```python
from build123d import *

# Parameters (mm, degrees)
CYLINDER062_R     = 1.25
CYLINDER062_DEPTH = 5
CYLINDER038_R     = 3
CYLINDER038_DEPTH = 4.1


with BuildPart() as b_w009:
    # Cylinder062 → Cylinder062 (new body)
    with BuildSketch(Plane(origin=(2, 6, 26), x_dir=(0, 0, 1), z_dir=(-1, 0, 0))):
        Circle(CYLINDER062_R)
    extrude(amount=CYLINDER062_DEPTH)


with BuildPart() as cut023:
    # Cylinder038 → Cylinder038 (new body)
    with BuildSketch(Plane(origin=(-1, 6, 26), x_dir=(0, 0, -1), z_dir=(1, 0, 0))):
        Circle(CYLINDER038_R)
    extrude(amount=CYLINDER038_DEPTH)

    # Cut023: cut B_W009
    add(b_w009.part, mode=Mode.SUBTRACT)


solid = cut023.part
```
CAD build for the part. Positions are in the model's coordinates, mm. Coordinates: 2 decimals unless noted, no trailing zeros. Order: outer loops, then holes, each group sorted by start corner. A loop starts at its lowest first (then second) coordinate and runs counter-clockwise, first axis right, second up. Notation, with made-up numbers: (55, -1) - (73, -1) arc R33 cw to (73, 37) - close; hole circle Ø7 at (-17.75, 53). An arc over 180 degrees is marked (long way). Use a Markdown table: item, result. Add a question column.
(1) Pull direction Y, two halves, no side cores. Call faces 1 (the face through (0.521, 5.521, 27.155)), 2 (the face through (2, 6, 26)), 3 (the face through (1, 4.2, 28.4)), 4 (the face through (-1, 5, 25)): +Y half, -Y half, draft (parallel to the pull), parting line (faces both ways), or undercut.
(2) Drill centre lines: line 1 along Y through (x, z) = (-0.2, 26); line 2 along Z through (x, y) = (0.95, 6.05); line 3 along X through (y, z) = (6, 26.7). Where is each one in solid material? Low to high. Write a range as [from, to].
(3) Saw through at D-D (y = 8). Give the cut face in (x, z).
(4) Saw through at B-B (y = 6). Give the cut face in (x, z).
(5) Flat gauge pins, fed straight in: pin 1 (2 mm diameter, centred on x = 0, z = 24.5, fed in from -Y); pin 2 (1.2 mm diameter, centred on y = 6, z = 25.5, fed in from -X); pin 3 (1.5 mm diameter, centred on x = 0, z = 27, fed in from +Y). Where does each tip first touch, or does it go through?
(6) Saw through at C-C (x = 0.55). Give the cut face in (y, z).
(7) Saw through at A-A (z = 26). Give the cut face in (x, y).
Solved:
| question | item | result |
|---|---|---|
| 1 | face 1 | undercut |
| 1 | face 2 | undercut |
| 1 | face 3 | parting line |
| 1 | face 4 | draft |
| 2 | line 1 | y = [3, 4.75], [7.25, 9] |
| 2 | line 2 | z = [23, 24.75], [27.25, 29] |
| 2 | line 3 | x = [2, 3.1] |
| 3 | outline | (-1, 23.76) - (3.1, 23.76) - (3.1, 28.24) - (-1, 28.24) - close |
| 4 | outline | (-1, 23) - (3.1, 23) - (3.1, 29) - (-1, 29) - (-1, 27.25) - (2, 27.25) - (2, 24.75) - (-1, 24.75) - close |
| 5 | pin 1 | stops at y = 3.04 |
| 5 | pin 2 | stops at x = 2 |
| 5 | pin 3 | stops at y = 8.99 |
| 6 | outline | circle Ø6 at (6, 26); hole circle Ø2.5 at (6, 26) |
| 7 | outline | (-1, 3) - (3.1, 3) - (3.1, 9) - (-1, 9) - (-1, 7.25) - (2, 7.25) - (2, 4.75) - (-1, 4.75) - close |
